Here's how the part is built. I have some questions about the finished solid (model axes, mm). A direction names the side the tool comes from. Coordinates: 2 decimals unless noted, no trailing zeros. Loops run counter-clockwise (first coordinate to the right, second up) from the corner with the lowest first, then second, coordinate; pieces in that order, holes last. Notation, with made-up numbers: (4, 87) -> (44, 87) arc R11 cw to (44, 105) -> close; hole circle Ø2 at (76.25, 87.5). An arc over 180 degrees is marked (long way). Answer as a JSON object with one key per item and string values. Group by question number.
Q1. I need wall thicknesses on line 1 (Z direction, x = 0, y = -21); line 2 (Y direction, x = 19, z = 19); line 3 (Z direction, x = 4.5, y = -13.5). Which ranges of each line are inside material? Lowest first, please.
Q2. Thinking about a two-plate mould opening in Z: for faces 1 (the flat face through (-24, -10, -30)), 2 (the flat face through (0, 0, 16)), 3 (the cylindrical face through (0.66, -13.366, 59.993)), 4 (the cylindrical face through (-2.17, -17.74, 20.24)), which applies, released by +Z, released by -Z, zero draft, split by the parting line, or undercut?
Q3. I want a section at D-D on x = 13. Write out the boundary of the cut face in (y, z), then the cut area to 3 significant figures.
Q4. I want a section at A-A on y = -6. Write out the boundary of the cut face in (x, z), then the cut area to 3 significant figures.
Q5. On a 3-axis mill with a long thin cutter (end or side, diameter ignored), from which of +Z, -Z, +X, -X, +Y, -Y can I reach the whole of each face in a straight line? I mean faces 5 (the flat face through (18, -27, 30)), 6 (the cylindrical face through (0, -27, 0)), 7 (the flat face through (-18, -27, 30)). Say none if no direction works.
Q6. I want a section at B-B on x = 0. Write out the boundary of the cut face in (y, z), then the cut area to 3 significant figures.
Q7. I want a section at C-C on z = 26. Write out the boundary of the cut face in (x, y).
Q8. I'm going to push flat-ended pins straight in: pin 1 (7.5 mm diameter, centred on y = -31, z = 33.5, fed in from +X); pin 2 (3 mm diameter, centred on y = -5, z = 43.5, fed in from -X); pin 3 (2 mm diameter, centred on x = 6, y = -6, fed in from +Z). Where does each tip first touch, or does it pass through?
```python
from build123d import *

# Parameters (mm, degrees)
F1_DEPTH = 20
F3_DEPTH = 15
F4_R     = 10
F5_DEPTH = 35.001


with BuildPart() as f1:
    # F0 (on Front) → F1 (new body)
    with BuildSketch(Plane.XZ):
        with BuildLine():
            Line((18, -30), (30, -30))
            Line((30, -30), (30, 30))
            ThreePointArc((30, 30), (0, 60), (-30, 30))
            Line((-30, 30), (-30, -30))
            Line((-30, -30), (-18, -30))
            ThreePointArc((-18, -30), (0, -12), (18, -30))
        make_face()
    extrude(amount=F1_DEPTH)

    # F2 (on face) → F3 (join)
    with BuildSketch(Plane.XZ.offset(20)):
        with BuildLine():
            Line((-18, 30), (-18, 6))
            ThreePointArc((-18, 6), (0, 0), (18, 6))
            Line((18, 6), (18, 30))
            Line((18, 30), (18, 54))
            ThreePointArc((18, 54), (0, 60), (-18, 54))
            Line((-18, 54), (-18, 30))
        make_face()
    extrude(amount=F3_DEPTH)

    # F4 (on face) → F5 (cut, through all)
    with BuildSketch(Plane.XZ.offset(35)):
        with Locations((0, 30)):
            Circle(F4_R)
    extrude(amount=-F5_DEPTH, mode=Mode.SUBTRACT)


solid = f1.part
```
Result set:
{
 "1": {"line 1": "z = 0 to 20, 40 to 60", "line 2": "y = -20 to 0", "line 3": "z = -12.57 to 21.07, 38.93 to 59.66"},
 "2": {"face 1": "released by -Z", "face 2": "zero draft", "face 3": "released by +Z", "face 4": "undercut"},
 "3": {"outline": "(-35, 2.96) -> (-20, 2.96) -> (-20, -17.55) -> (0, -17.55) -> (0, 57.04) -> (-35, 57.04) -> close", "area": "2,300 mm²"},
 "4": {"outline": "(-30, -30) -> (-18, -30) arc R18 cw to (18, -30) -> (30, -30) -> (30, 30) arc R30 ccw to (-30, 30) -> close; hole circle Ø20 at (0, 30)", "area": "4,190 mm²"},
 "5": {"face 5": "+Z, -Z, +X, -Y", "face 6": "-Z, -Y", "face 7": "+Z, -Z, -X, -Y"},
 "6": {"outline": "(-35, 0) -> (-20, 0) -> (-20, -12) -> (0, -12) -> (0, 20) -> (-35, 20) -> close; (-35, 40) -> (0, 40) -> (0, 60) -> (-35, 60) -> close", "area": "1,640 mm²"},
 "7": {"outline": "(-30, -20) -> (-18, -20) -> (-18, -35) -> (-9.17, -35) -> (-9.17, 0) -> (-30, 0) -> close; (9.17, -35) -> (18, -35) -> (18, -20) -> (30, -20) -> (30, 0) -> (9.17, 0) -> close"},
 "8": {"pin 1": "stops at x = 18", "pin 2": "stops at x = -27.5", "pin 3": "stops at z = 59.58"}
}
